Geometry check sheet. Reference: the model listing, model coordinates, mm. Round coordinates to 2 decimals unless told otherwise and drop trailing zeros. Loops run counter-clockwise (first coordinate to the right, second up) from the corner with the lowest first, then second, coordinate; pieces in that order, holes last. Notation, with made-up numbers: M -24,-30.75 L -3,-30.75 A21 cw -3,-17.75 Z; hole C 60.5,24.5 d9. An arc over 180 degrees is marked long. Write item = value, one per line.
from build123d import *

# Parameters (mm, degrees)
SKETCH_W                          = 16
SKETCH_H                          = 17
PAD_DEPTH                         = 1.6
SKETCH002_R                       = 0.41
POCKET_DEPTH                      = 48.401
POCKET_DEPTH_BACK                 = 46.801
SKETCH002_LINEARPATTERN_2_R       = 0.41
POCKET_LINEARPATTERN_2_DEPTH      = 48.401
POCKET_LINEARPATTERN_2_DEPTH_BACK = 46.801
SKETCH002_LINEARPATTERN_3_R       = 0.41
POCKET_LINEARPATTERN_3_DEPTH      = 48.401
POCKET_LINEARPATTERN_3_DEPTH_BACK = 46.801
SKETCH002_LINEARPATTERN_4_R       = 0.41
POCKET_LINEARPATTERN_4_DEPTH      = 48.401
POCKET_LINEARPATTERN_4_DEPTH_BACK = 46.801
SKETCH002_LINEARPATTERN_5_R       = 0.41
POCKET_LINEARPATTERN_5_DEPTH      = 48.401
POCKET_LINEARPATTERN_5_DEPTH_BACK = 46.801
SKETCH002_LINEARPATTERN_6_R       = 0.41
POCKET_LINEARPATTERN_6_DEPTH      = 48.401
POCKET_LINEARPATTERN_6_DEPTH_BACK = 46.801
SKETCH002_LINEARPATTERN_7_R       = 0.41
POCKET_LINEARPATTERN_7_DEPTH      = 48.401
POCKET_LINEARPATTERN_7_DEPTH_BACK = 46.801
SKETCH002_LINEARPATTERN_8_R       = 0.41
POCKET_LINEARPATTERN_8_DEPTH      = 48.401
POCKET_LINEARPATTERN_8_DEPTH_BACK = 46.801


with BuildPart() as part:
    # Sketch → Pad (new body)
    with BuildSketch(Plane.XZ):
        Rectangle(SKETCH_W, SKETCH_H)
    extrude(amount=PAD_DEPTH)

    # Sketch002 → Pocket (cut, two sides)
    with BuildSketch(Plane.XZ.offset(1.6)) as pocket_sk:
        with Locations((-8, 7)):
            Circle(SKETCH002_R)
    pocket = extrude(amount=-POCKET_DEPTH, mode=Mode.SUBTRACT) + extrude(pocket_sk.sketch, amount=POCKET_DEPTH_BACK, mode=Mode.SUBTRACT)

    # Sketch002 LinearPattern 2 → Pocket LinearPattern 2 (cut, two sides)
    with BuildSketch(Plane(origin=(0, -1.6, -2), x_dir=(1, 0, 0), z_dir=(0, -1, 0))) as pocket_linearpattern_2_sk:
        with Locations((-8, 7)):
            Circle(SKETCH002_LINEARPATTERN_2_R)
    pocket_linearpattern_2 = extrude(amount=-POCKET_LINEARPATTERN_2_DEPTH, mode=Mode.SUBTRACT) + extrude(pocket_linearpattern_2_sk.sketch, amount=POCKET_LINEARPATTERN_2_DEPTH_BACK, mode=Mode.SUBTRACT)

    # Sketch002 LinearPattern 3 → Pocket LinearPattern 3 (cut, two sides)
    with BuildSketch(Plane(origin=(0, -1.6, -4), x_dir=(1, 0, 0), z_dir=(0, -1, 0))) as pocket_linearpattern_3_sk:
        with Locations((-8, 7)):
            Circle(SKETCH002_LINEARPATTERN_3_R)
    pocket_linearpattern_3 = extrude(amount=-POCKET_LINEARPATTERN_3_DEPTH, mode=Mode.SUBTRACT) + extrude(pocket_linearpattern_3_sk.sketch, amount=POCKET_LINEARPATTERN_3_DEPTH_BACK, mode=Mode.SUBTRACT)

    # Sketch002 LinearPattern 4 → Pocket LinearPattern 4 (cut, two sides)
    with BuildSketch(Plane(origin=(0, -1.6, -6), x_dir=(1, 0, 0), z_dir=(0, -1, 0))) as pocket_linearpattern_4_sk:
        with Locations((-8, 7)):
            Circle(SKETCH002_LINEARPATTERN_4_R)
    pocket_linearpattern_4 = extrude(amount=-POCKET_LINEARPATTERN_4_DEPTH, mode=Mode.SUBTRACT) + extrude(pocket_linearpattern_4_sk.sketch, amount=POCKET_LINEARPATTERN_4_DEPTH_BACK, mode=Mode.SUBTRACT)

    # Sketch002 LinearPattern 5 → Pocket LinearPattern 5 (cut, two sides)
    with BuildSketch(Plane(origin=(0, -1.6, -8), x_dir=(1, 0, 0), z_dir=(0, -1, 0))) as pocket_linearpattern_5_sk:
        with Locations((-8, 7)):
            Circle(SKETCH002_LINEARPATTERN_5_R)
    pocket_linearpattern_5 = extrude(amount=-POCKET_LINEARPATTERN_5_DEPTH, mode=Mode.SUBTRACT) + extrude(pocket_linearpattern_5_sk.sketch, amount=POCKET_LINEARPATTERN_5_DEPTH_BACK, mode=Mode.SUBTRACT)

    # Sketch002 LinearPattern 6 → Pocket LinearPattern 6 (cut, two sides)
    with BuildSketch(Plane(origin=(0, -1.6, -10), x_dir=(1, 0, 0), z_dir=(0, -1, 0))) as pocket_linearpattern_6_sk:
        with Locations((-8, 7)):
            Circle(SKETCH002_LINEARPATTERN_6_R)
    pocket_linearpattern_6 = extrude(amount=-POCKET_LINEARPATTERN_6_DEPTH, mode=Mode.SUBTRACT) + extrude(pocket_linearpattern_6_sk.sketch, amount=POCKET_LINEARPATTERN_6_DEPTH_BACK, mode=Mode.SUBTRACT)

    # Sketch002 LinearPattern 7 → Pocket LinearPattern 7 (cut, two sides)
    with BuildSketch(Plane(origin=(0, -1.6, -12), x_dir=(1, 0, 0), z_dir=(0, -1, 0))) as pocket_linearpattern_7_sk:
        with Locations((-8, 7)):
            Circle(SKETCH002_LINEARPATTERN_7_R)
    pocket_linearpattern_7 = extrude(amount=-POCKET_LINEARPATTERN_7_DEPTH, mode=Mode.SUBTRACT) + extrude(pocket_linearpattern_7_sk.sketch, amount=POCKET_LINEARPATTERN_7_DEPTH_BACK, mode=Mode.SUBTRACT)

    # Sketch002 LinearPattern 8 → Pocket LinearPattern 8 (cut, two sides)
    with BuildSketch(Plane(origin=(0, -1.6, -14), x_dir=(1, 0, 0), z_dir=(0, -1, 0))) as pocket_linearpattern_8_sk:
        with Locations((-8, 7)):
            Circle(SKETCH002_LINEARPATTERN_8_R)
    pocket_linearpattern_8 = extrude(amount=-POCKET_LINEARPATTERN_8_DEPTH, mode=Mode.SUBTRACT) + extrude(pocket_linearpattern_8_sk.sketch, amount=POCKET_LINEARPATTERN_8_DEPTH_BACK, mode=Mode.SUBTRACT)

    # Mirrored: Pocket, Pocket LinearPattern 2, Pocket LinearPattern 3, Pocket LinearPattern 4, Pocket LinearPattern 5, Pocket LinearPattern 6, Pocket LinearPattern 7, Pocket LinearPattern 8 across YZ
    add(pocket.mirror(Plane.YZ), mode=Mode.SUBTRACT)
    add(pocket_linearpattern_2.mirror(Plane.YZ), mode=Mode.SUBTRACT)
    add(pocket_linearpattern_3.mirror(Plane.YZ), mode=Mode.SUBTRACT)
    add(pocket_linearpattern_4.mirror(Plane.YZ), mode=Mode.SUBTRACT)
    add(pocket_linearpattern_5.mirror(Plane.YZ), mode=Mode.SUBTRACT)
    add(pocket_linearpattern_6.mirror(Plane.YZ), mode=Mode.SUBTRACT)
    add(pocket_linearpattern_7.mirror(Plane.YZ), mode=Mode.SUBTRACT)
    add(pocket_linearpattern_8.mirror(Plane.YZ), mode=Mode.SUBTRACT)


solid = part.part
(1) Release check for a two-part mould opening along Z. For faces 1 (the flat face through (0, -1.6, 0)), 2 (the cylindrical face through (-7.59, -0.81, 2.99)), 3 (the cylindrical face through (-7.59, -0.81, 6.99)), 4 (the flat face through (0, -1, 8.5)) record: released by +Z, released by -Z, zero draft, split by the parting line, or undercut.
Result set:
face_1 = zero draft
face_2 = undercut
face_3 = undercut
face_4 = released by +Z
(2) Material ranges on line 1 along X through (y, z) = (-1.25, 7); line 2 along X through (y, z) = (-0.55, -1.25), recorded low to high. Write a range as from..to.
Result set:
line_1 = -7.59..7.59
line_2 = -7.68..7.68
(3) Sectioned sample at A-A on z = -1. Record the cut outline in (x, y), then the cut area to 3 significant figures.
Result set:
outline = M -7.59,-1.6 L 7.59,-1.6 L 7.59,0 L -7.59,0 Z
area = 24.3 mm2
